```python
from build123d import *

# Parameters (mm, degrees)
SKETCH_1_R          = 3
EXTRUDE_1_DEPTH     = 26
SKETCH_2_R          = 3
SKETCH_2_R_2        = 2.75
CUT_EXTRUDE_1_DEPTH = 0.35


with BuildPart() as part:
    # 스케치1 → 보스-돌출1 (new body)
    with BuildSketch(Plane.XY):
        with Locations(Location((0, 0, 0), (0, 0, 180))):
            Circle(SKETCH_1_R)
    extrude(amount=EXTRUDE_1_DEPTH)

    # 스케치2 → 컷-돌출1 (cut, symmetric)
    with BuildSketch(Plane(origin=(0, 0, 1.5), x_dir=(-1, 0, 0), z_dir=(0, 0, -1))):
        Circle(SKETCH_2_R)
        Circle(SKETCH_2_R_2, mode=Mode.SUBTRACT)
    cut_extrude_1 = extrude(amount=CUT_EXTRUDE_1_DEPTH, both=True, mode=Mode.SUBTRACT)

    # 대칭 복사1: 컷-돌출1 across plane
    add(cut_extrude_1.mirror(Plane(origin=(0, 0, 13), x_dir=(1, 0, 0), z_dir=(0, 0, -1))), mode=Mode.SUBTRACT)


solid = part.part
```
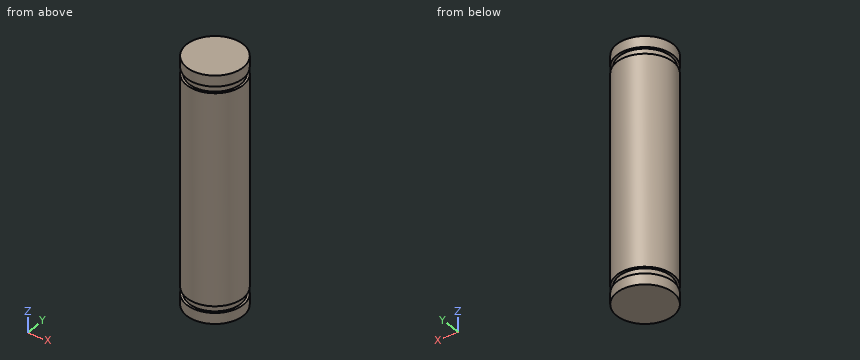
Part model, mm, in its own coordinate system. Round coordinates to 2 decimals unless told otherwise and drop trailing zeros. Write each loop counter-clockwise with the first axis right and the second up, starting at its lowest first coordinate (ties: lowest second). Pieces come first, ordered by that corner, then holes. Notation, with made-up numbers: M 47,51.25 L 95,51.25 A18 cw 95,60.25 Z; hole C -4,-1.5 d9. An arc over 180 degrees is marked long. One line per question, with ' | ' between items.
(1) Saw through at C-C on z = 3.75. Write the cut outline in (x, y).
Answer key:
outline: C 0,0 d6
(2) Saw through at A-A on x = -1.8. Write the cut outline in (y, z), then the cut area to 3 significant figures.
Answer key:
outline: M -2.4,0 L 2.4,0 L 2.4,1.15 L 2.08,1.15 L 2.08,1.85 L 2.4,1.85 L 2.4,24.15 L 2.08,24.15 L 2.08,24.85 L 2.4,24.85 L 2.4,26 L -2.4,26 L -2.4,24.85 L -2.08,24.85 L -2.08,24.15 L -2.4,24.15 L -2.4,1.85 L -2.08,1.85 L -2.08,1.15 L -2.4,1.15 Z | area: 124 mm^2
(3) Probe line 1 along Z through (x, y) = (2, 1.95); line 2 along Y through (x, z) = (0.9, 13.25); line 3 along Y through (x, z) = (-0.35, 25). List the from-to ranges inside material, lowest first.
Answer key:
line 1: z = 0 to 1.15, 1.85 to 24.15, 24.85 to 26 | line 2: y = -2.86 to 2.86 | line 3: y = -2.98 to 2.98
(4) Saw through at B-B on y = -1.9. Write the cut outline in (x, z).
Answer key:
outline: M -2.32,0 L 2.32,0 L 2.32,1.15 L 1.99,1.15 L 1.99,1.85 L 2.32,1.85 L 2.32,24.15 L 1.99,24.15 L 1.99,24.85 L 2.32,24.85 L 2.32,26 L -2.32,26 L -2.32,24.85 L -1.99,24.85 L -1.99,24.15 L -2.32,24.15 L -2.32,1.85 L -1.99,1.85 L -1.99,1.15 L -2.32,1.15 Z
